Here's how the part is built. I have some questions about the finished solid (model axes, mm). Face numbers are marked on the shaded views. A direction names the side the tool comes from. Round coordinates to 2 decimals unless told otherwise and drop trailing zeros. Order: outer loops, then holes, each group sorted by start corner. A loop starts at its lowest first (then second) coordinate and runs counter-clockwise, first axis right, second up. Notation, with made-up numbers: (45, 45.25) - (49, 45.25) arc R19 ccw to (49, 77.25) - close; hole circle Ø5 at (-7.75, 16.25). An arc over 180 degrees is marked (long way). One line per item, written item: value.
from build123d import *

# Parameters (mm, degrees)
BASE_FLANGE1_DEPTH       = 10
CUT_EXTRUDE1_REACH       = 27.713
MITER_START              = 3.625
MITER_FLANGE1_DEPTH      = 2.75
MITER_START_2            = 18.571970472
MITER_FLANGE4_DEPTH      = 4.220143907
MITER_START_3            = 17.844797598
MITER_FLANGE5_DEPTH      = 4.227172874
CUT_EXTRUDE8_DEPTH       = 0.727172875
CUT_EXTRUDE9_START       = -0.720143907
CUT_EXTRUDE9_DEPTH       = 0.720143907
CUT_EXTRUDE10_DEPTH      = 22.568364065
CUT_EXTRUDE10_DEPTH_BACK = 22.568364065
SKETCH26_W               = 10.008347653
SKETCH26_H               = 5.563663723


# Read off the part's stored shape, not the designer's step: Miter Flange1, Miter Flange4, Miter Flange5
# Sheet-metal steps are written as plain solids
with BuildPart() as part:
    # Sketch1 → Base-Flange1 (new body)
    with BuildSketch(Plane.XY):
        with BuildLine():
            Line((18.571970472, 61.565136218), (22.792114379, 61.565136218))
            ThreePointArc((22.792114379, 61.565136218), (22.964992643, 61.634545227), (23.041876434, 61.804231371))
            Line((23.041876434, 61.804231371), (23.061531352, 62.254403009))
            ThreePointArc((23.061531352, 62.254403009), (22.999729249, 62.43014431), (22.833558233, 62.51435653))
            Line((22.833558233, 62.51435653), (18.038908504, 62.933834027))
            ThreePointArc((18.038908504, 62.933834027), (17.856422666, 62.876296464), (17.768070893, 62.706574288))
            Line((17.768070893, 62.706574288), (17.595748923, 60.736925153))
            ThreePointArc((17.595748923, 60.736925153), (17.660478263, 60.546238666), (17.844797598, 60.465136218))
            Line((17.844797598, 60.465136218), (22.071970472, 60.465136218))
            Line((22.071970472, 60.465136218), (22.071970472, 60.065136218))
            Line((22.071970472, 60.065136218), (17.844797598, 60.065136218))
            ThreePointArc((17.844797598, 60.065136218), (17.365567329, 60.276002583), (17.197271044, 60.771787451))
            Line((17.197271044, 60.771787451), (17.369593014, 62.741436586))
            ThreePointArc((17.369593014, 62.741436586), (17.599307622, 63.182714241), (18.073770801, 63.332311907))
            Line((18.073770801, 63.332311907), (22.86842053, 62.91283441))
            ThreePointArc((22.86842053, 62.91283441), (23.300465172, 62.693882636), (23.461150641, 62.236955254))
            Line((23.461150641, 62.236955254), (23.441495723, 61.786783616))
            ThreePointArc((23.441495723, 61.786783616), (23.241597865, 61.345599642), (22.792114379, 61.165136218))
            Line((22.792114379, 61.165136218), (18.571970472, 61.165136218))
            Line((18.571970472, 61.165136218), (18.571970472, 61.565136218))
        make_face()
    extrude(amount=BASE_FLANGE1_DEPTH)

    # Sketch7 → Cut-Extrude1 (cut, up to next)
    with BuildSketch(Plane.XZ.offset(-60.065136218), mode=Mode.PRIVATE) as cut_extrude1_sk1:
        with BuildLine():
            Line((22.071970472, 3.375), (21.821970472, 3.375))
            ThreePointArc((21.821970472, 3.375), (21.696970472, 3.5), (21.821970472, 3.625))
            Line((21.821970472, 3.625), (22.071970472, 3.625))
            ThreePointArc((22.071970472, 3.625), (22.196970472, 3.5), (22.071970472, 3.375))
        make_face()
    cut_extrude1_tool1 = extrude(cut_extrude1_sk1.sketch, amount=-CUT_EXTRUDE1_REACH, mode=Mode.PRIVATE) & part.part
    # Sketch7 → Cut-Extrude1 (cut, up to next)
    with BuildSketch(Plane.XZ.offset(-60.065136218), mode=Mode.PRIVATE) as cut_extrude1_sk2:
        with BuildLine():
            Line((22.071970472, 6.375), (21.821970472, 6.375))
            ThreePointArc((21.821970472, 6.375), (21.696970472, 6.5), (21.821970472, 6.625))
            Line((21.821970472, 6.625), (22.071970472, 6.625))
            ThreePointArc((22.071970472, 6.625), (22.196970472, 6.5), (22.071970472, 6.375))
        make_face()
    cut_extrude1_tool2 = extrude(cut_extrude1_sk2.sketch, amount=-CUT_EXTRUDE1_REACH, mode=Mode.PRIVATE) & part.part
    add(cut_extrude1_tool1.solids().sort_by_distance((21.94697, 60.065136, 3.5))[0], mode=Mode.SUBTRACT)
    add(cut_extrude1_tool2.solids().sort_by_distance((21.94697, 60.065136, 6.5))[0], mode=Mode.SUBTRACT)

    # Miter Flange1 outline → Miter Flange1 (add)
    with BuildSketch(Plane.XY.offset(MITER_START)):
        with BuildLine():
            Line((22.321970472, 59.315136218), (22.721970472, 59.315136218))
            Line((22.721970472, 59.315136218), (22.721970472, 59.815136218))
            ThreePointArc((22.721970472, 59.815136218), (22.53158988, 60.274755626), (22.071970472, 60.465136218))
            Line((22.071970472, 60.465136218), (22.071970472, 60.065136218))
            ThreePointArc((22.071970472, 60.065136218), (22.248747167, 59.991912914), (22.321970472, 59.815136218))
            Line((22.321970472, 59.815136218), (22.321970472, 59.315136218))
        make_face()
    extrude(amount=MITER_FLANGE1_DEPTH)

    # Miter Flange4 outline → Miter Flange4 (add)
    with BuildSketch(Plane.YZ.offset(MITER_START_2)):
        with BuildLine():
            Line((61.99814892, 10.816987298), (61.651738758, 11.016987298))
            Line((61.651738758, 11.016987298), (61.252219705, 10.325))
            ThreePointArc((61.252219705, 10.325), (61.187284431, 10.168232379), (61.165136218, 10))
            Line((61.165136218, 10), (61.565136218, 10))
            ThreePointArc((61.565136218, 10), (61.573654761, 10.064704761), (61.598629867, 10.125))
            Line((61.598629867, 10.125), (61.99814892, 10.816987298))
        make_face()
    extrude(amount=MITER_FLANGE4_DEPTH)

    # Miter Flange5 outline → Miter Flange5 (add)
    with BuildSketch(Plane.YZ.offset(MITER_START_3)):
        with BuildLine():
            Line((59.978533677, 11.016987298), (59.632123516, 10.816987298))
            Line((59.632123516, 10.816987298), (60.031642569, 10.125))
            ThreePointArc((60.031642569, 10.125), (60.056617674, 10.064704761), (60.065136218, 10))
            Line((60.065136218, 10), (60.465136218, 10))
            ThreePointArc((60.465136218, 10), (60.442988005, 10.168232379), (60.37805273, 10.325))
            Line((60.37805273, 10.325), (59.978533677, 11.016987298))
        make_face()
    extrude(amount=MITER_FLANGE5_DEPTH)

    # Sketch20 → Cut-Extrude8 (cut)
    with BuildSketch(Plane.ZY.offset(-17.844797598)):
        with BuildLine():
            Line((10.125, 60.031642569), (10.816987298, 59.632123516))
            Line((10.816987298, 59.632123516), (11.016987298, 59.978533677))
            Line((11.016987298, 59.978533677), (10.325, 60.37805273))
            ThreePointArc((10.325, 60.37805273), (10.168232379, 60.442988005), (10, 60.465136218))
            Line((10, 60.465136218), (10, 60.065136218))
            ThreePointArc((10, 60.065136218), (10.064704761, 60.056617674), (10.125, 60.031642569))
        make_face()
    extrude(amount=-CUT_EXTRUDE8_DEPTH, mode=Mode.SUBTRACT)

    # Sketch23 → Cut-Extrude9 (cut)
    with BuildSketch(Plane(origin=(22.792114379, 0, 0), x_dir=(0, 0, -1), z_dir=(1, 0, 0)).offset(CUT_EXTRUDE9_START)):
        with BuildLine():
            Line((-10.125, 61.598629867), (-10.816987298, 61.99814892))
            Line((-10.816987298, 61.99814892), (-11.016987298, 61.651738758))
            Line((-11.016987298, 61.651738758), (-10.325, 61.252219705))
            ThreePointArc((-10.325, 61.252219705), (-10.168232379, 61.187284431), (-10, 61.165136218))
            Line((-10, 61.165136218), (-10, 61.565136218))
            ThreePointArc((-10, 61.565136218), (-10.064704761, 61.573654761), (-10.125, 61.598629867))
        make_face()
    extrude(amount=CUT_EXTRUDE9_DEPTH, mode=Mode.SUBTRACT)

    # Sketch26 → Cut-Extrude10 (cut, two sides: drawn at the far end of the back side and taken through both)
    with BuildSketch(Plane(origin=(5.63606087, 64.420470526, 0), x_dir=(0.9961946980917451, -0.08715574274766313, 0), z_dir=(0.08715574274766313, 0.9961946980917451, 0)).offset(-CUT_EXTRUDE10_DEPTH_BACK)):
        with Locations((14.807454486, -2.218168138)):
            Rectangle(SKETCH26_W, SKETCH26_H)
    extrude(amount=CUT_EXTRUDE10_DEPTH + CUT_EXTRUDE10_DEPTH_BACK, mode=Mode.SUBTRACT)

    # Mirror1: part across plane


with BuildPart() as part_1:
    add(part.part)
    add(part.part.mirror(Plane(origin=(25.016835548, 58.630796571, 5), x_dir=(1, 0, 0), z_dir=(0, 0, 1))))


solid = part_1.part
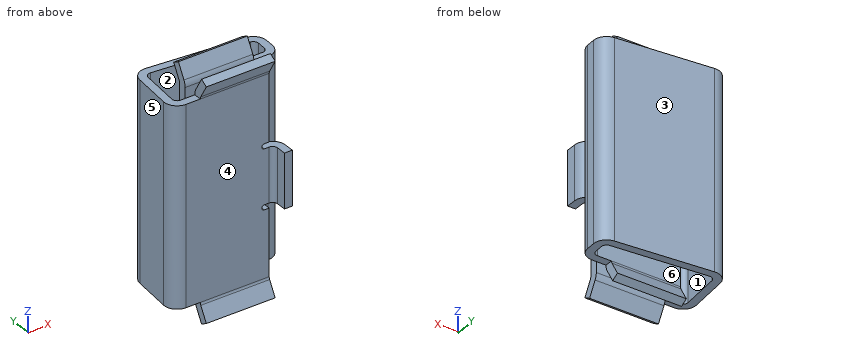
Q1. If we section it at C-C, the plane y = 60.95: Please give me the cut outline in (x, z).
Results list:
outline: (17.21, 0) - (17.61, 0) - (17.61, 10) - (17.21, 10) - close
Q2. Which directions (+Z, -Z, +X, -X, +Y, -Y) give clear straight access to the entire face, cutting with the end or side of a thin tool? Please do the marked faces 5 and 6.
Results list:
face 5: +Z, -Z, -X, +Y
face 6: none
Q3. If we section it at D-D, the plane z = 3.5: Please give me the cut outline in (x, y), then the cut area to 3 significant figures.
Results list:
outline: (17.2, 60.77) arc R0.65 ccw to (17.84, 60.07) - (21.7, 60.07) - (21.7, 60.47) - (17.84, 60.47) arc R0.25 cw to (17.6, 60.74) - (17.77, 62.71) arc R0.25 cw to (18.04, 62.93) - (22.83, 62.51) arc R0.25 cw to (23.06, 62.25) - (23.04, 61.8) arc R0.25 cw to (22.79, 61.57) - (18.57, 61.57) - (18.57, 61.17) - (22.79, 61.17) arc R0.65 ccw to (23.44, 61.79) - (23.46, 62.24) arc R0.65 ccw to (22.87, 62.91) - (18.07, 63.33) arc R0.65 ccw to (17.37, 62.74) - close
area: 7.26 mm²
Q4. If we section it at A-A, the plane x = 19.75: Please give me the cut outline in (y, z) (3 decimals), then the cut area to 3 significant figures.
Results list:
outline: (59.632, -0.817) - (59.979, -1.017) - (60.378, -0.325) arc R0.65 ccw to (60.465, 0) - (60.465, 10) arc R0.65 ccw to (60.378, 10.325) - (59.979, 11.017) - (59.632, 10.817) - (60.032, 10.125) arc R0.25 cw to (60.065, 10) - (60.065, 0) arc R0.25 cw to (60.032, -0.125) - close; (61.165, 0) arc R0.65 ccw to (61.252, -0.325) - (61.652, -1.017) - (61.998, -0.817) - (61.599, -0.125) arc R0.25 cw to (61.565, 0) - (61.565, 10) arc R0.25 cw to (61.599, 10.125) - (61.998, 10.817) - (61.652, 11.017) - (61.252, 10.325) arc R0.65 ccw to (61.165, 10) - close; (62.784, 0) - (63.186, 0) - (63.186, 10) - (62.784, 10) - close
area: 13.7 mm²
Q5. We'd pull the mould along Y, two halves only. Please class the marked faces 1, 2, 3 and 4: released by +Y, released by -Y, zero draft, split by the parting line, or undercut.
Results list:
face 1: undercut
face 2: undercut
face 3: released by +Y
face 4: released by -Y
Q6. If we section it at B-B, the plane z = 8: Please give me the cut outline in (x, y).
Results list:
outline: (17.2, 60.77) arc R0.65 ccw to (17.84, 60.07) - (22.07, 60.07) - (22.07, 60.47) - (17.84, 60.47) arc R0.25 cw to (17.6, 60.74) - (17.77, 62.71) arc R0.25 cw to (18.04, 62.93) - (22.83, 62.51) arc R0.25 cw to (23.06, 62.25) - (23.04, 61.8) arc R0.25 cw to (22.79, 61.57) - (18.57, 61.57) - (18.57, 61.17) - (22.79, 61.17) arc R0.65 ccw to (23.44, 61.79) - (23.46, 62.24) arc R0.65 ccw to (22.87, 62.91) - (18.07, 63.33) arc R0.65 ccw to (17.37, 62.74) - close
Q7. If I drill on line 1 along Y through (x, z) = (21.25, 9.5); line 2 along Y through (x, z) = (20, 1.5); line 3 along Y through (x, z) = (18.5, 6.25), over which ranges is the centre line in solid material (lowest first)?
Results list:
line 1: 60.07 to 60.47, 61.17 to 61.57, 62.65 to 63.05
line 2: 60.07 to 60.47, 61.17 to 61.57, 62.76 to 63.16
line 3: 60.07 to 60.47, 62.89 to 63.3
Q8. Will these pins go through, and if not, where does the flat tip stop? pin 1 (0.9 mm diameter, centred on y = 61.5, z = -0.5, fed in from +X); pin 2 (3.5 mm diameter, centred on x = 20.5, z = 4.5, fed in from +Y); pin 3 (1.6 mm diameter, centred on x = 20.5, y = 61.5, fed in from -Z).
Results list:
pin 1: x = 22.07
pin 2: y = 63.27
pin 3: z = -1.02
